Part print with two shaded views. Sizes in mm from the minimum x, y, z corner. A direction names the side the tool comes from. Give positions to 0.01 mm unless a question says otherwise; leave off trailing zeros. Loops run counter-clockwise (first coordinate to the right, second up) from the corner with the lowest first, then second, coordinate; pieces in that order, holes last. Notation, with made-up numbers: M 89,-40 L 110,-40 A34 ccw 110,-6 Z; hole C 20,-13 d1. An arc over 180 degrees is marked long. Answer in a Markdown table with one row per item.
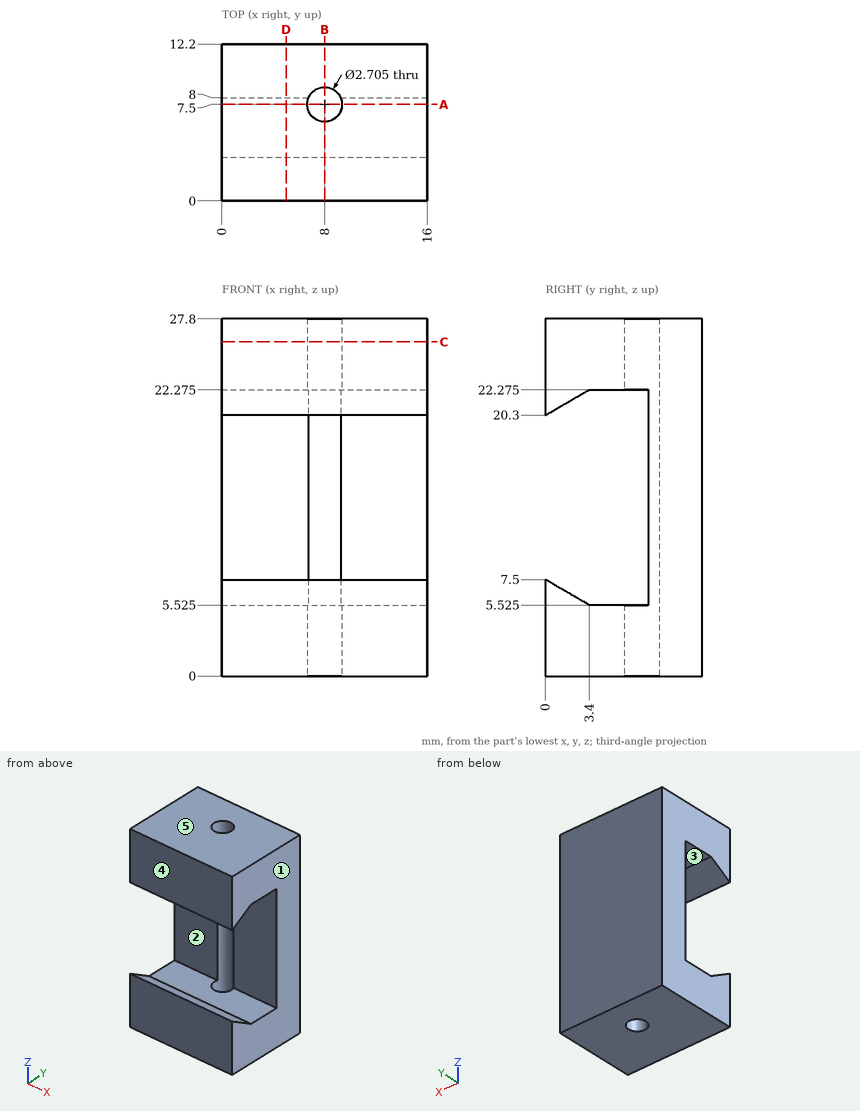
Q1. Saw through at D-D (x = 5). Give the cut face in (y, z) (3 decimals).
Reported:
| item | result |
|---|---|
| outline | M 0,0 L 12.2,0 L 12.2,27.8 L 0,27.8 L 0,20.3 L 3.4,22.275 L 8,22.275 L 8,5.525 L 3.4,5.525 L 0,7.5 Z |
Q2. Saw through at C-C (z = 26). Give the cut face in (x, y) (1 decimal).
Reported:
| item | result |
|---|---|
| outline | M 0,0 L 16,0 L 16,12.2 L 0,12.2 Z; hole C 8,7.5 d2.7 |
Q3. Probe probe 1 along Z at (x, y) = (8.75, 6.25) (3 decimals); probe 2 along Y at (x, z) = (8, 14.75); probe 3 along Y at (x, z) = (2, 6.5). List the from-to ranges inside material, lowest first.
Reported:
| item | result |
|---|---|
| probe 1 | 0 to 5.525, 22.275 to 27.8 |
| probe 2 | 8.85 to 12.2 |
| probe 3 | 0 to 1.72, 8 to 12.2 |
Q4. Saw through at B-B (x = 8). Give the cut face in (y, z) (1 decimal).
Reported:
| item | result |
|---|---|
| outline | M 0,0 L 6.1,0 L 6.1,5.5 L 3.4,5.5 L 0,7.5 Z; M 0,20.3 L 3.4,22.3 L 6.1,22.3 L 6.1,27.8 L 0,27.8 Z; M 8.9,0 L 12.2,0 L 12.2,27.8 L 8.9,27.8 Z |
Q5. 3-axis set-ups, long thin cutter, end or side, ignore diameter. For the marked faces 1 and 2: which of +Z, -Z, +X, -X, +Y, -Y reach the whole face in a straight line?
Reported:
| item | result |
|---|---|
| face 1 | +Z, -Z, +X, +Y, -Y |
| face 2 | +X, -X |
Q6. Saw through at A-A (y = 7.5). Give the cut face in (x, z) (1 decimal).
Reported:
| item | result |
|---|---|
| outline | M 0,0 L 6.6,0 L 6.6,5.5 L 0,5.5 Z; M 0,22.3 L 6.6,22.3 L 6.6,27.8 L 0,27.8 Z; M 9.4,0 L 16,0 L 16,5.5 L 9.4,5.5 Z; M 9.4,22.3 L 16,22.3 L 16,27.8 L 9.4,27.8 Z |
Q7. Drop a flat-ended pin along its axis: pin 1 (5.5 mm diameter, centred on x = 11.5, z = 15, fed in from -Y). Give the stop position or say it passes through.
Reported:
| item | result |
|---|---|
| pin 1 | y = 8 |
Q8. Mould opens along Y. For the marked faces 3, 4 and 5 say: released by +Y, released by -Y, zero draft, split by the parting line, or undercut.
Reported:
| item | result |
|---|---|
| face 3 | undercut |
| face 4 | released by -Y |
| face 5 | zero draft |
